Can you work these out from the model? Positions are in its coordinate system, mm. Face numbers are marked on the shaded views. A direction names the side the tool comes from. Round coordinates to 2 decimals unless told otherwise and drop trailing zeros. Write each loop counter-clockwise with the first axis right and the second up, starting at its lowest first coordinate (ties: lowest second). Pieces come first, ordered by that corner, then holes. Notation, with made-up numbers: M 25.25,40.5 L 82.25,40.5 A23 cw 82.25,68.5 Z; hole C 21.25,0 d4. An arc over 180 degrees is marked long. Answer as a JSON object with one key per item and string values. Group by question number.
1) If we mould it in two halves opening along X, with no side actions, what happens to the marked faces 4, 5 and 6? For each: +X half, -X half, draft (parallel to the pull), parting line (faces both ways), or undercut.
2) I'm going to push flat-ended pins straight in: pin 1 Ø3 at (x, y) = (-28.5, -6.5) entering from +Z; pin 2 Ø3 at (x, z) = (1.5, -2) entering from -Y; pin 3 Ø1.5 at (y, z) = (-11, 1) entering from +X. Where does each tip first touch, or does it pass through?
3) Suppose I cut it at C-C, the plane y = -12. Write out the boundary of the cut face in (x, z), and give its area (3 significant figures).
4) Suppose I cut it at A-A, the plane x = 27.1. Write out the boundary of the cut face in (y, z), and give its area (3 significant figures).
5) On a 3-axis mill with a long thin cutter (end or side, diameter ignored), from which of +Z, -Z, +X, -X, +Y, -Y can I reach the whole of each face in a straight line? I mean the marked faces 1, 2 and 3. Say none if no direction works.
6) Please list where these lines run through material, in increasing order: L1, parallel to X at y = -8, z = -6; L2, parallel to X at y = -14, z = -0.25; L3, parallel to X at y = -5.5, z = 4.75. Write a range as [from, to].
7) Suppose I cut it at B-B, the plane z = -5.25. Write out the boundary of the cut face in (x, y), and give its area (3 significant figures).
8) Suppose I cut it at D-D, the plane z = 0.25. Write out the boundary of the cut face in (x, y).
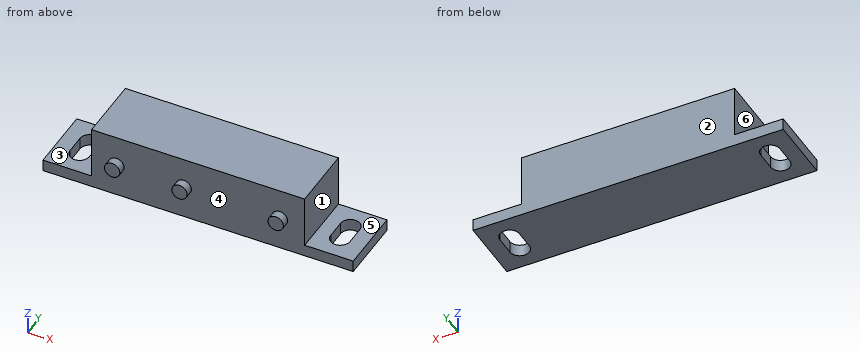
from build123d import *

# Parameters (mm, degrees)
F0_W     = 64.5
F0_H     = 13.5
F1_DEPTH = 13.6
F2_W     = 10.1
F2_H     = 13.6
F3_DEPTH = 11
F4_R     = 1.6
F5_DEPTH = 1.7
F7_DEPTH = 25


with BuildPart() as f1:
    # F0 (on Front) → F1 (new body)
    with BuildSketch(Plane.XZ):
        Rectangle(F0_W, F0_H)
    extrude(amount=F1_DEPTH)

    # F2 (on face) → F3 (cut)
    with BuildSketch(Plane.XY.offset(6.75)):
        with Locations((-27.2, -6.8)):
            Rectangle(F2_W, F2_H)
        with Locations((27.2, -6.8)):
            Rectangle(F2_W, F2_H)
    extrude(amount=-F3_DEPTH, mode=Mode.SUBTRACT)

    # F4 (on face) → F5 (join)
    with BuildSketch(Plane.XZ.offset(13.6)):
        with Locations((17, 0.25)):
            Circle(F4_R)
        with Locations((-3, 0.25)):
            Circle(F4_R)
        with Locations((-17, 0.25)):
            Circle(F4_R)
    extrude(amount=F5_DEPTH)

    # F6 (on face) → F7 (cut)
    with BuildSketch(Plane.XY.offset(-4.25)):
        with BuildLine():
            ThreePointArc((-25.1, -4.8), (-27.1, -2.8), (-29.1, -4.8))
            Line((-29.1, -4.8), (-29.1, -6.8))
            Line((-29.1, -6.8), (-29.1, -8.8))
            ThreePointArc((-29.1, -8.8), (-27.1, -10.8), (-25.1, -8.8))
            Line((-25.1, -8.8), (-25.1, -6.8))
            Line((-25.1, -6.8), (-25.1, -4.8))
        make_face()
        with BuildLine():
            Line((29.1, -8.8), (29.1, -4.8))
            ThreePointArc((29.1, -4.8), (27.1, -2.8), (25.1, -4.8))
            Line((25.1, -4.8), (25.1, -8.8))
            ThreePointArc((25.1, -8.8), (27.1, -10.8), (29.1, -8.8))
        make_face()
    extrude(amount=-F7_DEPTH, mode=Mode.SUBTRACT)


solid = f1.part
Results:
{
 "1": {"face 4": "undercut", "face 5": "draft", "face 6": "-X half"},
 "2": {"pin 1": "z = -4.25", "pin 2": "y = -13.6", "pin 3": "x = 22.15"},
 "3": {"outline": "M -32.25,-6.75 L 32.25,-6.75 L 32.25,-4.25 L 22.15,-4.25 L 22.15,6.75 L -22.15,6.75 L -22.15,-4.25 L -32.25,-4.25 Z", "area": "649 mm^2"},
 "4": {"outline": "M -13.6,-6.75 L -10.8,-6.75 L -10.8,-4.25 L -13.6,-4.25 Z; M -2.8,-6.75 L 0,-6.75 L 0,-4.25 L -2.8,-4.25 Z", "area": "14.0 mm^2"},
 "5": {"face 1": "+Z, +X, +Y, -Y", "face 2": "+Z, -Z, +X, -X, +Y", "face 3": "+Z, -X, +Y, -Y"},
 "6": {"L1": "[-32.25, -29.1], [-25.1, 25.1], [29.1, 32.25]", "L2": "[-18.52, -15.48], [-4.52, -1.48], [15.48, 18.52]", "L3": "[-22.15, 22.15]"},
 "7": {"outline": "M -32.25,-13.6 L 32.25,-13.6 L 32.25,0 L -32.25,0 Z; hole M -29.1,-8.8 A2 ccw -25.1,-8.8 L -25.1,-4.8 A2 ccw -29.1,-4.8 Z; hole M 25.1,-8.8 A2 ccw 29.1,-8.8 L 29.1,-4.8 A2 ccw 25.1,-4.8 Z", "area": "820 mm^2"},
 "8": {"outline": "M -22.15,-13.6 L -18.6,-13.6 L -18.6,-15.3 L -15.4,-15.3 L -15.4,-13.6 L -4.6,-13.6 L -4.6,-15.3 L -1.4,-15.3 L -1.4,-13.6 L 15.4,-13.6 L 15.4,-15.3 L 18.6,-15.3 L 18.6,-13.6 L 22.15,-13.6 L 22.15,0 L -22.15,0 Z"}
}
